Geometry check sheet. Reference: the model listing, model coordinates, mm. A direction names the side the tool comes from. Coordinates: 2 decimals unless noted, no trailing zeros. Order: outer loops, then holes, each group sorted by start corner. A loop starts at its lowest first (then second) coordinate and runs counter-clockwise, first axis right, second up. Notation, with made-up numbers: (8.25, 15.5) -> (58.25, 15.5) arc R34 cw to (58.25, 52.5) -> close; hole circle Ø2 at (78.25, 49). An arc over 180 degrees is marked (long way). Answer as CSV lines item,"result". Start each with the question number.
from build123d import *

# Parameters (mm, degrees)
ESQUISSE1_R                     = 17.7
ESQUISSE1_R_2                   = 12.7
BOSS_EXTRU_1_DEPTH              = 8.7
ESQUISSE2_R                     = 30.4
ESQUISSE2_R_2                   = 11.2
BOSS_EXTRU_2_DEPTH              = 47.8
CHANFREIN1_SIZE                 = 25.4
CHANFREIN1_SIZE2                = 12.699971641
CHANFREIN3_SIZE                 = 11.200084029
CHANFREIN3_SIZE_2               = 49.8
F_41_0_096_DIAMETER_HOLE1_D     = 2.4384
F_41_0_096_DIAMETER_HOLE1_DEPTH = 5
F_41_0_096_DIAMETER_HOLE1_TIP   = 0.732569267


with BuildPart() as part:
    # Esquisse1 → Boss.-Extru.1 (new body)
    with BuildSketch(Plane.XY):
        Circle(ESQUISSE1_R)
        Circle(ESQUISSE1_R_2, mode=Mode.SUBTRACT)
    extrude(amount=BOSS_EXTRU_1_DEPTH)

    # Esquisse2 → Boss.-Extru.2 (add)
    with BuildSketch(Plane(origin=(0, 0, 0), x_dir=(-1, 0, 0), z_dir=(0, 0, -1))):
        with Locations(Location((0, 0, 0), (0, 0, 180))):
            Circle(ESQUISSE2_R)
        with Locations(Location((0, 0, 0), (0, 0, 180))):
            Circle(ESQUISSE2_R_2, mode=Mode.SUBTRACT)
    extrude(amount=BOSS_EXTRU_2_DEPTH)

    # Chanfrein1
    chanfrein1_edges = [part.edges().sort_by_distance(p)[0] for p in [
        (-30.4, 0, 0),
    ]]
    chanfrein1_side = [part.faces().sort_by_distance(p)[0] for p in [
        (-30.4, 0, -23.9),
    ]]
    chamfer(chanfrein1_edges, length=CHANFREIN1_SIZE, length2=CHANFREIN1_SIZE2, reference=chanfrein1_side[0])

    # Chanfrein3
    # the kernel refuses this chamfer: 49.8, 11.200084029 mm, written as the material it takes off along each edge
    with BuildSketch(Plane(origin=(0, 0, -47.8), x_dir=(1, 0, 0), z_dir=(0, 1, 0))) as chanfrein3_piece_1:
        Polygon((11.2 + CHANFREIN3_SIZE, 0), (11.2, -CHANFREIN3_SIZE_2), (11.2, 0), align=None)
    revolve(axis=Axis((0, 0, -47.8), (0, 0, -1)), mode=Mode.SUBTRACT)

    # #41 (0.096) Diameter Hole1
    with Locations(Plane.XY.offset(8.7)):
        with Locations((-15.2, 0), (15.2, 0)):
            Hole(F_41_0_096_DIAMETER_HOLE1_D / 2, depth=F_41_0_096_DIAMETER_HOLE1_DEPTH)
            with Locations((0, 0, -(F_41_0_096_DIAMETER_HOLE1_DEPTH + F_41_0_096_DIAMETER_HOLE1_TIP / 2))):  # 118° drill point
                Cone(0, F_41_0_096_DIAMETER_HOLE1_D / 2, F_41_0_096_DIAMETER_HOLE1_TIP, mode=Mode.SUBTRACT)


solid = part.part
Q1. Sectioned sample at B-B, the plane z = -33. Record the cut outline in (x, y), then the cut area to 3 significant figures.
Q2. Go/stop test with flat-tipped pins: pin 1 Ø3 at (x, z) = (-22.5, -15.5) entering from -Y; pin 2 Ø4 at (y, z) = (-11, -12) entering from -X; pin 3 Ø8 at (y, z) = (-3, -19) entering from -X; pin 4 Ø7.5 at (x, y) = (-1.5, -4.5) entering from +Z. Record where each tip stops, or that it passes through.
Q3. Release check for a two-part mould opening along Y. For faces 1 (the flat face through (-14, 18, -47.8)), 2 (the cylindrical face through (16.88, 5.32, 4.29)), 3 (the cylindrical face through (-2.75, -12.4, 4.29)) record: released by +Y, released by -Y, zero draft, split by the parting line, or undercut.
Q4. Sectioned sample at C-C, the plane z = -15. Record the cut outline in (x, y).
Q5. Thickness scan on L1, parallel to Y at x = 0, z = 5; L2, parallel to Y at x = 15.2, z = 5.75; L3, parallel to X at y = 1.5, z = 1.5. Record the ranges inside material, lowest first.
Q6. Access from +Z, -Z, +X, -X, +Y, -Y to the whole of each face (thin tool, end or side, straight path). Record for faces 4 (the cylindrical face through (14.04, 0.37, 6.16)), 5 (the conical face through (15.028, -4.732, -18.254)).
Geometry results:
1,outline,"circle Ø60.8 at (0, 0); hole circle Ø38.14 at (0, 0)"
1,area,"1,760 mm^2"
2,pin 1,"stops at y = -14.75"
2,pin 2,"stops at x = -22.46"
2,pin 3,"stops at x = -29.08"
2,pin 4,"passes through"
3,face 1,"zero draft"
3,face 2,"split by the parting line"
3,face 3,"undercut"
4,outline,"circle Ø50.4 at (0, 0); hole circle Ø30.05 at (0, 0)"
5,L1,"y = -17.7 to -12.7, 12.7 to 17.7"
5,L2,"y = -9.07 to -1.22, 1.22 to 9.07"
5,L3,"x = -17.64 to -12.61, 12.61 to 17.64"
6,face 4,"+Z"
6,face 5,"-Z"
